```python
from build123d import *

# Parameters (mm, degrees)
BOSS_EXTRUDE1_DEPTH = 40
BOSS_EXTRUDE2_DEPTH = 5
LPATTERN1_COUNT     = 2
LPATTERN1_PITCH     = 10
SKETCH4_R           = 1.5
CUT_EXTRUDE2_DEPTH  = 91.293964361


# Read off the part's stored shape, not the designer's step: Mirror1
with BuildPart() as part:
    # Sketch1 → Boss-Extrude1 (new body)
    with BuildSketch(Plane(origin=(0, 0, 0), x_dir=(0, 0, -1), z_dir=(1, 0, 0))):
        Polygon((0, 0), (0, 23), (9, 23), (9, 0), (6.2, 0), (6.2, 20), (2.8, 20), (2.8, 0), align=None)
    extrude(amount=BOSS_EXTRUDE1_DEPTH)

    # Sketch3 → Boss-Extrude2 (add)
    with BuildSketch(Plane.ZY):
        with BuildLine():
            Line((0, 0), (28, 0))
            Line((28, 0), (28, 5))
            ThreePointArc((28, 5), (6.132470247, 15.132470247), (-4, 37))
            Line((-4, 37), (-4, 72))
            Line((-4, 72), (-9, 72))
            Line((-9, 72), (-9, 37))
            Line((-9, 37), (-9, 23))
            Line((-9, 23), (0, 23))
            Line((0, 23), (0, 0))
        make_face()
    boss_extrude2 = extrude(amount=-BOSS_EXTRUDE2_DEPTH)

    # LPattern1: Boss-Extrude2 ×2
    with Locations(*[(i * LPATTERN1_PITCH, 0, 0) for i in range(1, LPATTERN1_COUNT)]):
        add(boss_extrude2)

    # Sketch4 → Cut-Extrude2 (cut, through all)
    with BuildSketch(Plane(origin=(0, 0, -9), x_dir=(-1, 0, 0), z_dir=(0, 0, -1))):
        with Locations(Location((-10, 10, 0), (0, 0, 270))):
            Circle(SKETCH4_R)
        with Locations(Location((-20, 10, 0), (0, 0, 90))):
            Circle(SKETCH4_R)
        with Locations(Location((-30, 10, 0), (0, 0, 90))):
            Circle(SKETCH4_R)
    extrude(amount=-CUT_EXTRUDE2_DEPTH, mode=Mode.SUBTRACT)

    # Mirror1: part across plane


with BuildPart() as part_1:
    add(part.part)
    add(part.part.mirror(Plane.ZY.offset(-20)))


solid = part_1.part
```
Verification items for the finished model (mm, model axes). A direction names the side the tool comes from. Coordinates: 2 decimals unless noted, no trailing zeros. Write each loop counter-clockwise with the first axis right and the second up, starting at its lowest first coordinate (ties: lowest second). Pieces come first, ordered by that corner, then holes. Notation, with made-up numbers: M 14.25,38 L 25.25,38 A17 ccw 25.25,57 Z; hole C -34,-27.5 d6. An arc over 180 degrees is marked long. One line per item, written item: value.
Item 1: Scan lines: line 1 along X through (y, z) = (10, 6.5); line 2 along Z through (x, y) = (9.5, 18); line 3 along X through (y, z) = (10, -1.55). Record each from-to range of solid material in increasing order.
Check sheet entries:
line 1: x = 0 to 5, 11.5 to 15, 25 to 28.5, 35 to 40
line 2: z = -9 to -6.2, -2.8 to 0
line 3: x = 0 to 8.5, 11.5 to 18.5, 21.5 to 28.5, 31.5 to 40
Item 2: Section check B-B, the plane y = 42. Record the boundary of the cut face in (x, z), plus the area to 3 significant figures.
Check sheet entries:
outline: M 0,-9 L 5,-9 L 5,-4 L 0,-4 Z; M 10,-9 L 15,-9 L 15,-4 L 10,-4 Z; M 25,-9 L 30,-9 L 30,-4 L 25,-4 Z; M 35,-9 L 40,-9 L 40,-4 L 35,-4 Z
area: 100 mm^2
Item 3: Mould release check, pull along X, two halves, no side actions. Record for faces 1 (the flat face through (35, 28, -3)), 2 (the flat face through (33, 23, -4)), 3 (the flat face through (0, 23, -2)), 4 (the flat face through (38, 2, 28)): pulls with the +X half, pulls with the -X half, needs draft (parallel to the pull), parting line crosses it, or undercut.
Check sheet entries:
face 1: undercut
face 2: undercut
face 3: pulls with the -X half
face 4: needs draft
Item 4: Section check A-A, the plane x = 20. Record the boundary of the cut face in (y, z), plus the area to 3 significant figures.
Check sheet entries:
outline: M 0,-9 L 8.5,-9 L 8.5,-6.2 L 0,-6.2 Z; M 0,-2.8 L 8.5,-2.8 L 8.5,0 L 0,0 Z; M 11.5,-9 L 23,-9 L 23,0 L 11.5,0 L 11.5,-2.8 L 20,-2.8 L 20,-6.2 L 11.5,-6.2 Z
area: 122 mm^2
Item 5: Section check C-C, the plane z = 19.5. Record the boundary of the cut face in (x, y), plus the area to 3 significant figures.
Check sheet entries:
outline: M 0,0 L 5,0 L 5,6.78 L 0,6.78 Z; M 10,0 L 15,0 L 15,6.78 L 10,6.78 Z; M 25,0 L 30,0 L 30,6.78 L 25,6.78 Z; M 35,0 L 40,0 L 40,6.78 L 35,6.78 Z
area: 136 mm^2
Item 6: Section check D-D, the plane x = 37. Record the boundary of the cut face in (y, z), plus the area to 3 significant figures.
Check sheet entries:
outline: M 0,-9 L 72,-9 L 72,-4 L 37,-4 A35 cw 5,28 L 0,28 L 0,-2.8 L 20,-2.8 L 20,-6.2 L 0,-6.2 Z
area: 707 mm^2
Item 7: Gauge pin test, flat ends, axial feed: pin 1 Ø2.5 at (x, y) = (3, 57) entering from +Z; pin 2 Ø1.5 at (x, z) = (8, -5) entering from +Y; pin 3 Ø4 at (x, y) = (30, 34.5) entering from +Z; pin 4 Ø2 at (x, y) = (32, 29) entering from -Z. Record the tip position at first contact, or that the pin passes through.
Check sheet entries:
pin 1: stops at z = -4
pin 2: stops at y = 23
pin 3: stops at z = -3.33
pin 4: passes through
Item 8: Access from +Z, -Z, +X, -X, +Y, -Y to the whole of each face (thin tool, end or side, straight path). Record for faces 5 (the flat face through (20, 20, -5)), 6 (the flat face through (10, 4, 14)), 7 (the flat face through (38, 54, -4)).
Check sheet entries:
face 5: +X, -X, -Y
face 6: +Z, +Y, -Y
face 7: +Z, +X, -X, +Y
